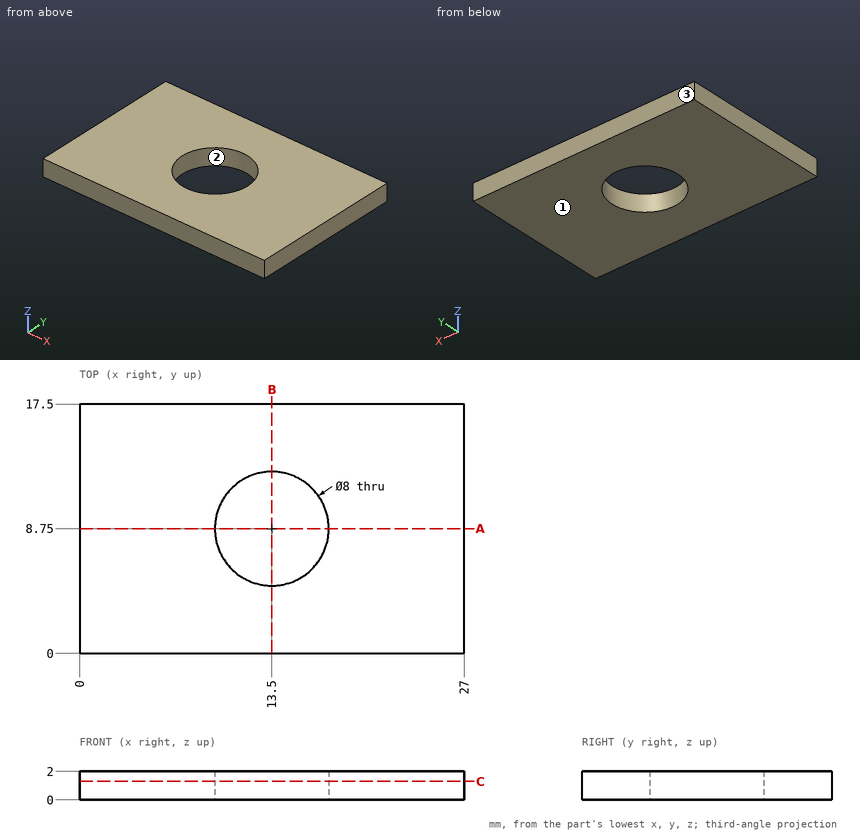
Study the drawing (mm; zero at the part's minimum x, y, z) and answer. Give positions to 0.01 mm unless a question says otherwise; leave off trailing zeros. Write each loop counter-clockwise with the first axis right and the second up, starting at its lowest first coordinate (ties: lowest second). Pieces come first, ordered by that corner, then holes. Notation, with made-up numbers: (79.25, 4.25) - (97.25, 4.25) arc R23 ccw to (97.25, 17.25) - close; hole circle Ø8 at (64.25, -27). An arc over 180 degrees is marked (long way). Write item = value, one per line. Start each with the question number.
Item 1: This flat-tipped pin is pushed along its axis until it touches: P1, Ø7, axis at x = 13.5, y = 8.75, coming from the +Z side. Where does it stop, or does it pass through?
Item 2: Find section C-C (z = 1.3). Give the vertices of the cut face in (x, y), then the cut area to 3 significant figures.
Item 3: Find section B-B (x = 13.5). Give the vertices of the cut face in (y, z), then the cut area to 3 significant figures.
Item 4: Find the intervals of material crossed by probe 1 along Y at (x, z) = (13.5, 1.5); probe 2 along X at (y, z) = (9, 0.75); probe 3 along X at (y, z) = (11, 1.3), in increasing order. Write a range as [from, to].
Item 5: Find section A-A (y = 8.75). Give the vertices of the cut face in (x, z).
Item 6: The mould has two halves that part along Y. Classify the marked faces 1, 2 and 3: +Y half, -Y half, draft (parallel to the pull), parting line (faces both ways), or undercut.
Response:
q1.P1 = through
q2.outline = (0, 0) - (27, 0) - (27, 17.5) - (0, 17.5) - close; hole circle Ø8 at (13.5, 8.75)
q2.area = 422 mm²
q3.outline = (0, 0) - (4.75, 0) - (4.75, 2) - (0, 2) - close; (12.75, 0) - (17.5, 0) - (17.5, 2) - (12.75, 2) - close
q3.area = 19.0 mm²
q4.probe_1 = [0, 4.75], [12.75, 17.5]
q4.probe_2 = [0, 9.51], [17.49, 27]
q4.probe_3 = [0, 10.19], [16.81, 27]
q5.outline = (0, 0) - (9.5, 0) - (9.5, 2) - (0, 2) - close; (17.5, 0) - (27, 0) - (27, 2) - (17.5, 2) - close
q6.face_1 = draft
q6.face_2 = undercut
q6.face_3 = +Y half
